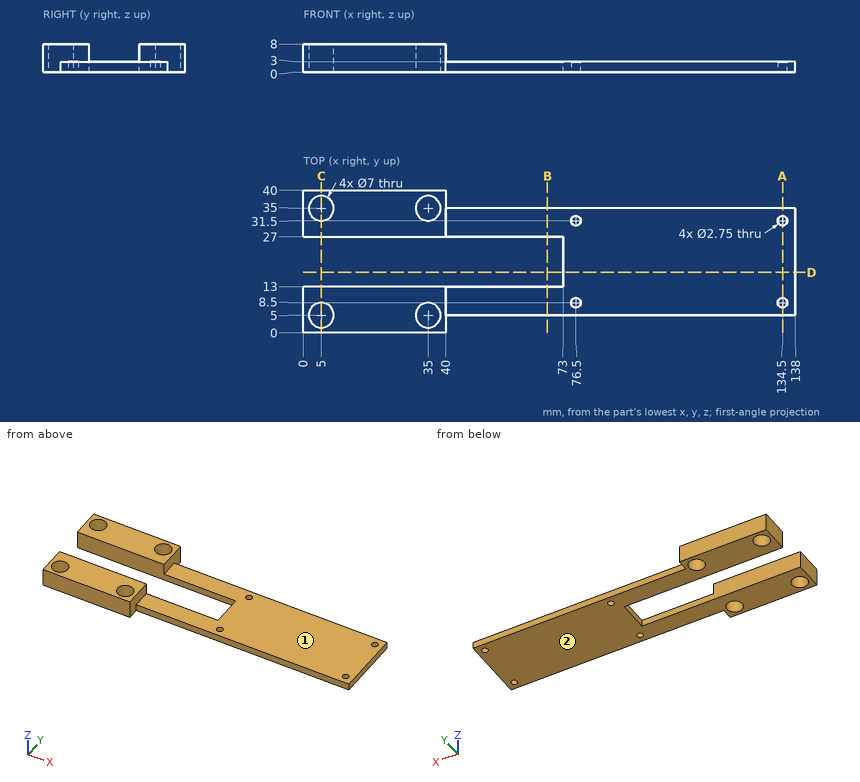
Drawing for the job (mm, zero at the part's lowest x, y, z). A direction names the side the tool comes from. Coordinates: 2 decimals unless noted, no trailing zeros. Order: outer loops, then holes, each group sorted by start corner. A loop starts at its lowest first (then second) coordinate and runs counter-clockwise, first axis right, second up. Notation, with made-up numbers: (7, 65.5) -> (22, 65.5) arc R28 cw to (22, 89.5) -> close; hole circle Ø3 at (40, -39). An arc over 180 degrees is marked (long way). One line per item, written item: value.
(1) Tool access for the marked faces 1 and 2: list every direction of +Z, -Z, +X, -X, +Y, -Y with a clear straight run to the whole face (end or side of a thin tool).
Checked values:
face 1: +Z, +X, +Y, -Y
face 2: -Z, +X, -X, +Y, -Y
(2) Drop flat-ended pins along their axis: pin 1 Ø2.5 at (y, z) = (4, 4.5) entering from +X; pin 2 Ø4.5 at (x, y) = (76.5, 31.5) entering from +Z; pin 3 Ø6.5 at (x, y) = (5, 35) entering from -Z; pin 4 Ø2.5 at (x, z) = (98, 1) entering from +Y. Give the stop position or say it passes through.
Checked values:
pin 1: x = 40
pin 2: z = 3
pin 3: through
pin 4: y = 35
(3) Slice it at D-D, the plane y = 17. List the corners of the cut face in (x, z), plus the area to 3 significant figures.
Checked values:
outline: (73, 0) -> (138, 0) -> (138, 3) -> (73, 3) -> close
area: 195 mm2
(4) Slice it at B-B, the plane x = 68.5. List the corners of the cut face in (y, z).
Checked values:
outline: (5, 0) -> (13, 0) -> (13, 3) -> (5, 3) -> close; (27, 0) -> (35, 0) -> (35, 3) -> (27, 3) -> close
(5) Slice it at C-C, the plane x = 5. List the corners of the cut face in (y, z), plus the area to 3 significant figures.
Checked values:
outline: (0, 0) -> (1.5, 0) -> (1.5, 8) -> (0, 8) -> close; (8.5, 0) -> (13, 0) -> (13, 8) -> (8.5, 8) -> close; (27, 0) -> (31.5, 0) -> (31.5, 8) -> (27, 8) -> close; (38.5, 0) -> (40, 0) -> (40, 8) -> (38.5, 8) -> close
area: 96.0 mm2
(6) Probe line 1 (Y direction, x = 5, z = 2.75); line 2 (Y direction, x = 76.5, z = 1.7) (3 decimals); line 3 (Y direction, x = 9, z = 2.5). List the from-to ranges inside material, lowest first. Write a range as [from, to].
Checked values:
line 1: [0, 1.5], [8.5, 13], [27, 31.5], [38.5, 40]
line 2: [5, 7.125], [9.875, 30.125], [32.875, 35]
line 3: [0, 13], [27, 40]
(7) Slice it at A-A, the plane x = 134.5. List the corners of the cut face in (y, z) (3 decimals).
Checked values:
outline: (5, 0) -> (7.125, 0) -> (7.125, 3) -> (5, 3) -> close; (9.875, 0) -> (30.125, 0) -> (30.125, 3) -> (9.875, 3) -> close; (32.875, 0) -> (35, 0) -> (35, 3) -> (32.875, 3) -> close
